CAD build for the part. Positions are in the model's coordinates, mm. A direction names the side the tool comes from. Round coordinates to 2 decimals unless told otherwise and drop trailing zeros. Order: outer loops, then holes, each group sorted by start corner. A loop starts at its lowest first (then second) coordinate and runs counter-clockwise, first axis right, second up. Notation, with made-up numbers: M 72,-9.5 L 108,-9.5 A30 cw 108,15.5 Z; hole C -18,-39 d1. An arc over 180 degrees is marked long. Answer as CSV lines item,"result". Start each with the question number.
```python
from build123d import *

# Parameters (mm, degrees)
SKETCH_1_R      = 29.5
EXTRUDE_1_DEPTH = 20
SKETCH_3_R      = 10
EXTRUDE_2_DEPTH = 300
SKETCH_4_R      = 29.5
EXTRUDE_3_DEPTH = 20
FILLET_1_R      = 1


with BuildPart() as part:
    # 草图1 → 凸台-拉伸1 (new body)
    with BuildSketch(Plane.XZ.offset(-1690.101215638)):
        with Locations(Location((0, 0, 0), (0, 0, 270))):
            Circle(SKETCH_1_R)
    extrude(amount=-EXTRUDE_1_DEPTH)

    # 草图3 → 凸台-拉伸2 (add)
    with BuildSketch(Plane(origin=(0, 1710.101215638, 0), x_dir=(1, 0, 0), z_dir=(0, 1, 0))):
        with Locations(Location((0, 0, 0), (0, 0, 270))):
            Circle(SKETCH_3_R)
    extrude(amount=EXTRUDE_2_DEPTH)

    # 草图4 → 凸台-拉伸3 (add)
    with BuildSketch(Plane(origin=(0, 2010.101215638, 0), x_dir=(1, 0, 0), z_dir=(0, 1, 0))):
        with Locations(Location((0, 0, 0), (0, 0, 90))):
            Circle(SKETCH_4_R)
    extrude(amount=EXTRUDE_3_DEPTH)

    # 圆角1
    fillet_1_edges = [part.edges().sort_by_distance(p)[0] for p in [
        (0, 1710.101215638, -10),
        (0, 2010.101215638, -10),
    ]]
    fillet(fillet_1_edges, radius=FILLET_1_R)


solid = part.part
```
Q1. Band-saw the part on D-D, the plane z = 0. Write the cut outline in (x, y).
Q2. Tool access for faces 4 (the cylindrical face through (-8.86, 2019.96, -28.14)), 5 (the flat face through (0, 1710.101, -13)): list every direction of +Z, -Z, +X, -X, +Y, -Y with a clear straight run to the whole face (end or side of a thin tool).
Q3. Drop flat-ended pins along their axis: P1, Ø10, axis at y = 1992, z = -13.5, coming from the +X side; P2, Ø1, axis at x = 1, y = 1842, coming from the -Z side; P3, Ø3, axis at y = 1865.5, z = -3.5, coming from the -X side. Give the stop position or say it passes through.
Q4. Probe line 1 along Y through (x, z) = (21, 6.5); line 2 along X through (y, z) = (2013.5, 2); line 3 along X through (y, z) = (1839.5, 1). List the from-to ranges inside material, lowest first. Write a range as from..to.
Q5. Band-saw the part on B-B, the plane z = -16. Write the cut outline in (x, y).
Q6. Band-saw the part on C-C, the plane x = 22. Write the cut outline in (y, z).
Q7. Band-saw the part on A-A, the plane x = 0. Write the cut outline in (y, z).
Q8. Mould opens along Y. For faces 1 (the flat face through (0, 1690.101, 0)), 2 (the cylindrical face through (-9.76, 1858.02, -2.17)), 3 (the flat face through (0, 2030.101, 0)) say: +Y half, -Y half, draft (parallel to the pull), parting line (faces both ways), or undercut.
Answer:
1,outline,"M -29.5,1690.1 L 29.5,1690.1 L 29.5,1710.1 L 11,1710.1 A1 cw 10,1711.1 L 10,2009.1 A1 cw 11,2010.1 L 29.5,2010.1 L 29.5,2030.1 L -29.5,2030.1 L -29.5,2010.1 L -11,2010.1 A1 cw -10,2009.1 L -10,1711.1 A1 cw -11,1710.1 L -29.5,1710.1 Z"
2,face 4,"+Y, -Y"
2,face 5,"none"
3,P1,"stops at x = 5.27"
3,P2,"stops at z = -9.99"
3,P3,"stops at x = -9.8"
4,line 1,"y = 1690.1..1710.1, 2010.1..2030.1"
4,line 2,"x = -29.43..29.43"
4,line 3,"x = -9.95..9.95"
5,outline,"M -24.78,1690.1 L 24.78,1690.1 L 24.78,1710.1 L -24.78,1710.1 Z; M -24.78,2010.1 L 24.78,2010.1 L 24.78,2030.1 L -24.78,2030.1 Z"
6,outline,"M 1690.1,-19.65 L 1710.1,-19.65 L 1710.1,19.65 L 1690.1,19.65 Z; M 2010.1,-19.65 L 2030.1,-19.65 L 2030.1,19.65 L 2010.1,19.65 Z"
7,outline,"M 1690.1,-29.5 L 1710.1,-29.5 L 1710.1,-11 A1 cw 1711.1,-10 L 2009.1,-10 A1 cw 2010.1,-11 L 2010.1,-29.5 L 2030.1,-29.5 L 2030.1,29.5 L 2010.1,29.5 L 2010.1,11 A1 cw 2009.1,10 L 1711.1,10 A1 cw 1710.1,11 L 1710.1,29.5 L 1690.1,29.5 Z"
8,face 1,"-Y half"
8,face 2,"undercut"
8,face 3,"+Y half"
